Verification items for the finished model (mm, model axes). Face numbers are marked on the shaded views. Coordinates: 2 decimals unless noted, no trailing zeros. Order: outer loops, then holes, each group sorted by start corner. A loop starts at its lowest first (then second) coordinate and runs counter-clockwise, first axis right, second up. Notation, with made-up numbers: M 49.5,35.25 L 94.5,35.25 A23 ccw 94.5,73.25 Z; hole C 48.5,-37 d10. An arc over 180 degrees is marked long. Return JSON: item names as keys, results as strings. Group by question number.
Q1. Section check A-A, the plane x = 0. Enter the section's corners in (y, z).
Q2. Section check B-B, the plane y = 0. Enter the section's corners in (x, z).
Q3. Go/stop test with flat-tipped pins: pin 1 Ø8 at (x, z) = (24, 43.5) entering from -Y; pin 2 Ø8 at (x, z) = (47.5, 39.5) entering from -Y; pin 3 Ø1.5 at (y, z) = (15.5, 30) entering from -X. Record where each tip stops, or that it passes through.
Q4. Thickness scan on probe 1 along X at (y, z) = (25.5, 7); probe 2 along X at (y, z) = (0, 23); probe 3 along X at (y, z) = (-27.5, 24.5). Record the ranges inside material, lowest first.
Q5. Section check C-C, the plane z = 18. Enter the section's corners in (x, y).
Q6. Mould release check, pull along X, two halves, no side actions. Record for the marked faces 1 and 2: pulls with the +X half, pulls with the -X half, needs draft (parallel to the pull), parting line crosses it, or undercut.
from build123d import *

# Parameters (mm, degrees)
F1_DEPTH = 50.8


# Not quite as in the source:
# - the program builds the solid bodies; features that only make, move or delete a surface that nothing else refers to are left out


with BuildPart() as f1:
    # F0 (on Top) → F1 (new body)
    with BuildSketch(Plane.XY):
        with BuildLine():
            ThreePointArc((71.697641485, 22.5322768092), (57.8335915966, 38.0459789198), (40.8652917128, 26.0058945539))
            ThreePointArc((40.8652917128, 26.0058945539), (49.8001603414, 18.2709960085), (53.6773841191, 7.1073197012))
            ThreePointArc((53.6773841191, 7.1073197012), (66.2378886043, 10.6720599339), (71.697641485, 22.5322768092))
        make_face()
        with BuildLine():
            ThreePointArc((40.8652917128, 26.0058945539), (29.7902072309, 28.2756215729), (18.9821024809, 24.9598971069))
            ThreePointArc((18.9821024809, 24.9598971069), (28.094084627, 13.9297913535), (31.3578806392, 0))
            ThreePointArc((31.3578806392, 0), (30.0861647392, -8.8396475875), (26.3741656765, -16.9623130219))
            ThreePointArc((26.3741656765, -16.9623130219), (45.3624091415, -12.2385728556), (53.7378936923, 5.4452720199))
            ThreePointArc((53.7378936923, 5.4452720199), (53.7227612897, 6.2768464158), (53.6773841191, 7.1073197012))
            ThreePointArc((53.6773841191, 7.1073197012), (43.1635782705, 13.7717941683), (40.8652917128, 26.0058945539))
        make_face()
        with BuildLine():
            ThreePointArc((53.6773841191, 7.1073197012), (49.8001603414, 18.2709960085), (40.8652917128, 26.0058945539))
            ThreePointArc((40.8652917128, 26.0058945539), (43.1635782705, 13.7717941683), (53.6773841191, 7.1073197012))
        make_face()
        with BuildLine():
            ThreePointArc((25.2208191949, -16.6990878355), (28.9640451764, -8.7197099962), (30.2481281305, 0))
            ThreePointArc((30.2481281305, 0), (27.0098398624, 13.6168207012), (17.9883409986, 24.3180764765))
            ThreePointArc((17.9883409986, 24.3180764765), (8.3723071222, 1.4762729148), (25.2208191949, -16.6990878355))
        make_face()
        with BuildLine():
            ThreePointArc((17.9883409986, 24.3180764765), (27.0098398624, 13.6168207012), (30.2481281305, 0))
            ThreePointArc((30.2481281305, 0), (28.9640451764, -8.7197099962), (25.2208191949, -16.6990878355))
            ThreePointArc((25.2208191949, -16.6990878355), (25.7957891487, -16.8381635446), (26.3741656765, -16.9623130219))
            ThreePointArc((26.3741656765, -16.9623130219), (30.0861647392, -8.8396475875), (31.3578806392, 0))
            ThreePointArc((31.3578806392, 0), (28.094084627, 13.9297913535), (18.9821024809, 24.9598971069))
            ThreePointArc((18.9821024809, 24.9598971069), (18.4810686237, 24.6454172593), (17.9883409986, 24.3180764765))
        make_face()
        with BuildLine():
            ThreePointArc((25.2208191949, -16.6990878355), (-29.7885854516, -5.2525643445), (17.9883409986, 24.3180764765))
            ThreePointArc((17.9883409986, 24.3180764765), (18.4810686237, 24.6454172593), (18.9821024809, 24.9598971069))
            ThreePointArc((18.9821024809, 24.9598971069), (-30.881478119, -5.4452720199), (26.3741656765, -16.9623130219))
            ThreePointArc((26.3741656765, -16.9623130219), (25.7957891487, -16.8381635446), (25.2208191949, -16.6990878355))
        make_face()
        with BuildLine():
            ThreePointArc((25.2208191949, -16.6990878355), (8.3723071222, 1.4762729148), (17.9883409986, 24.3180764765))
            ThreePointArc((17.9883409986, 24.3180764765), (-29.7885854516, -5.2525643445), (25.2208191949, -16.6990878355))
        make_face()
    extrude(amount=F1_DEPTH)


solid = f1.part
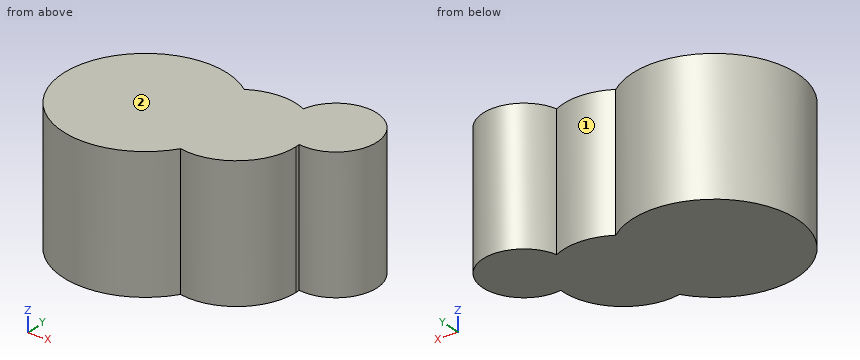
Numbers:
{
 "1": {"outline": "M -31.36,0 L 31.36,0 L 31.36,50.8 L -31.36,50.8 Z"},
 "2": {"outline": "M -31.36,0 L 53.08,0 L 53.08,50.8 L -31.36,50.8 Z"},
 "3": {"pin 1": "stops at y = -24.15", "pin 2": "stops at y = -13.61", "pin 3": "stops at x = -27.67"},
 "4": {"probe 1": "x = -18.25 to 18.25, 19.92 to 71.41", "probe 2": "x = -31.36 to 53.08", "probe 3": "x = -15.07 to 15.07"},
 "5": {"outline": "M 18.98,24.96 A31.36 ccw long 26.37,-16.96 A22.86 ccw 53.68,7.11 A15.61 ccw long 40.87,26.01 A22.86 ccw Z"},
 "6": {"face 1": "undercut", "face 2": "needs draft"}
}
